For this review, take the finished solid that the model builds, in its own axes (mm). A direction names the side the tool comes from. Round coordinates to 2 decimals unless told otherwise and drop trailing zeros. Order: outer loops, then holes, each group sorted by start corner. A loop starts at its lowest first (then second) coordinate and runs counter-clockwise, first axis right, second up. Notation, with made-up numbers: (39.5, 56) - (89.5, 56) arc R17 ccw to (89.5, 70) - close; hole circle Ø1 at (79, 20). An arc over 180 degrees is marked (long way). One line per item, written item: value.
```python
from build123d import *

# Parameters (mm, degrees)
SKETCH1_W               = 9.525
SKETCH1_H               = 19.05
BOSS_EXTRUDE1_DEPTH     = 12.7
BOSS_EXTRUDE2_DEPTH     = 50.8
CUT_EXTRUDE1_DEPTH      = 114.668287772
CUT_EXTRUDE1_DEPTH_BACK = 114.668287772


with BuildPart() as part:
    # Sketch1 → Boss-Extrude1 (new body)
    with BuildSketch(Plane.XY):
        with Locations((32.7025, 4.948874545)):
            Rectangle(SKETCH1_W, SKETCH1_H)
    extrude(amount=-BOSS_EXTRUDE1_DEPTH)

    # Sketch2 → Boss-Extrude2 (add)
    with BuildSketch(Plane(origin=(0, 14.473874545, 0), x_dir=(1, 0, 0), z_dir=(0, 1, 0))):
        with BuildLine():
            ThreePointArc((46.582827663, 71.746075344), (42.767883123, 83.788084157), (32.714892878, 91.436689602))
            ThreePointArc((32.714892878, 91.436689602), (0, 97.112987913), (-32.714892878, 91.436689602))
            ThreePointArc((-32.714892878, 91.436689602), (-42.767883123, 83.788084157), (-46.582827663, 71.746075344))
            Line((-46.582827663, 71.746075344), (-46.582827663, 68.977736354))
            Line((-46.582827663, 68.977736354), (-37.465, 12.7))
            Line((-37.465, 12.7), (-27.94, 12.7))
            Line((-27.94, 12.7), (-35.072238217, 70.222747392))
            ThreePointArc((-35.072238217, 70.222747392), (-30.65501556, 79.862333542), (-20.059817821, 79.443690492))
            ThreePointArc((-20.059817821, 79.443690492), (-17.502300297, 78.909892112), (-15.410312677, 80.474955814))
            ThreePointArc((-15.410312677, 80.474955814), (-9.316307054, 85.127912481), (-1.767954793, 83.782814559))
            ThreePointArc((-1.767954793, 83.782814559), (0, 83.245040535), (1.767954793, 83.782814559))
            ThreePointArc((1.767954793, 83.782814559), (9.316307054, 85.127912481), (15.410312677, 80.474955814))
            ThreePointArc((15.410312677, 80.474955814), (17.502300297, 78.909892112), (20.059817821, 79.443690492))
            ThreePointArc((20.059817821, 79.443690492), (29.98783501, 80.23610137), (35.194839749, 71.746075344))
            Line((35.194839749, 71.746075344), (35.194839749, 62.905769869))
            Line((35.194839749, 62.905769869), (27.94, 12.7))
            Line((27.94, 12.7), (37.465, 12.7))
            Line((37.465, 12.7), (46.582827663, 68.977736354))
            Line((46.582827663, 68.977736354), (46.582827663, 71.746075344))
        make_face()
    extrude(amount=-BOSS_EXTRUDE2_DEPTH)

    # Sketch3 → Cut-Extrude1 (cut, two sides: drawn at the far end of the back side and taken through both)
    with BuildSketch(Plane(origin=(0, 0, 0), x_dir=(0, 0, -1), z_dir=(1, 0, 0)).offset(-CUT_EXTRUDE1_DEPTH_BACK)):
        Polygon((80.788094726, -36.326125455), (12.7, -4.576125455), (12.7, -36.326125455), align=None)
        Polygon((97.112987913, -24.888548166), (12.7, 14.473874545), (97.112987913, 14.473874545), align=None)
    extrude(amount=CUT_EXTRUDE1_DEPTH + CUT_EXTRUDE1_DEPTH_BACK, mode=Mode.SUBTRACT)


solid = part.part
```
Item 1: Machinability: for faces 1 (the flat face through (37.465, 5, -6)), 2 (the flat face through (31.618, -6.46, -38.154)), 3 (the cylindrical face through (42.9, -27.1, -83.6)), which of the approach directions +Z, -Z, +X, -X, +Y, -Y give a long, thin tool a straight path to every point of the face, cutting with its end or side? Answer none if there is none.
Returned:
face 1: +Z, +X, +Y, -Y
face 2: +Y, -Y
face 3: -Z, +X, +Y, -Y
Item 2: Take a section at C-C (z = -57). Write out the cut boundary in (x, y), plus the area to 3 significant figures.
Returned:
outline: (-44.64, -25.23) - (-33.43, -25.23) - (-33.43, -6.18) - (-44.64, -6.18) - close; (34.34, -25.23) - (44.64, -25.23) - (44.64, -6.18) - (34.34, -6.18) - close
area: 410 mm^2
Item 3: Take a section at B-B (y = 3). Write out the cut boundary in (x, z) (1 decimal), plus the area to 3 significant figures.
Returned:
outline: (-41.5, -37.3) - (-31, -37.3) - (-27.9, -12.7) - (-37.5, -12.7) - close; (27.9, -12.7) - (31.5, -37.3) - (41.5, -37.3) - (37.5, -12.7) - (37.5, 0) - (27.9, 0) - close
area: 607 mm^2
Item 4: For P1, Ø5, axis at x = -33, y = 4.5, coming from the +Z side; P2, Ø5, axis at x = 34, z = -9.5, coming from the -Y side; P3, Ø4, axis at y = -13.5, z = -29, coming from the +X side, all flat-tipped, find the tip position at first contact; note any pin that passes through.
Returned:
P1: z = -12.7
P2: y = -4.58
P3: x = 40.42
Item 5: Take a section at A-A (z = -43.5). Write out the cut boundary in (x, y), plus the area to 3 significant figures.
Returned:
outline: (-42.46, -18.94) - (-31.76, -18.94) - (-31.76, 0.11) - (-42.46, 0.11) - close; (32.39, -18.94) - (42.46, -18.94) - (42.46, 0.11) - (32.39, 0.11) - close
area: 395 mm^2
Item 6: The part is to be moulded in two halves that separate along Z. For faces 4 (the flat face through (-33, 5, -12.7)), 5 (the flat face through (35.195, -20, -67)), 6 (the flat face through (33, -4.576, -6)), say which applies: +Z half, -Z half, draft (parallel to the pull), parting line (faces both ways), or undercut.
Returned:
face 4: +Z half
face 5: undercut
face 6: draft
Item 7: Wall thickness on line 1 (Y direction, x = -35.5, z = -69); line 2 (X direction, y = -2.5, z = -25); line 3 (Y direction, x = -35.5, z = -57): over which ranges is each line inside the solid? List them lowest first.
Returned:
line 1: -30.83 to -11.78
line 2: -39.46 to -29.47, 29.72 to 39.46
line 3: -25.23 to -6.18
Item 8: Take a section at D-D (y = -23.5). Write out the cut boundary in (x, z) (3 decimals), plus the area to 3 significant figures.
Returned:
outline: (-46.583, -71.746) arc R20.913 ccw to (-32.715, -91.437) arc R97.113 ccw to (-23.864, -94.135) - (23.864, -94.135) arc R97.113 ccw to (32.715, -91.437) arc R20.913 ccw to (46.583, -71.746) - (46.583, -68.978) - (44.04, -53.282) - (33.804, -53.282) - (35.195, -62.906) - (35.195, -71.746) arc R9.525 cw to (20.06, -79.444) arc R3.175 ccw to (15.41, -80.475) arc R9.525 cw to (1.768, -83.783) arc R3.175 ccw to (-1.768, -83.783) arc R9.525 cw to (-15.41, -80.475) arc R3.175 ccw to (-20.06, -79.444) arc R9.525 cw to (-35.072, -70.223) - (-32.972, -53.282) - (-44.04, -53.282) - (-46.583, -68.978) - close
area: 1,550 mm^2
